Geometry check sheet. Reference: drawing and pictorial views, mm from the part's lowest x, y, z. Give positions to 0.01 mm unless a question says otherwise; leave off trailing zeros. Order: outer loops, then holes, each group sorted by start corner. A loop starts at its lowest first (then second) coordinate and runs counter-clockwise, first axis right, second up.
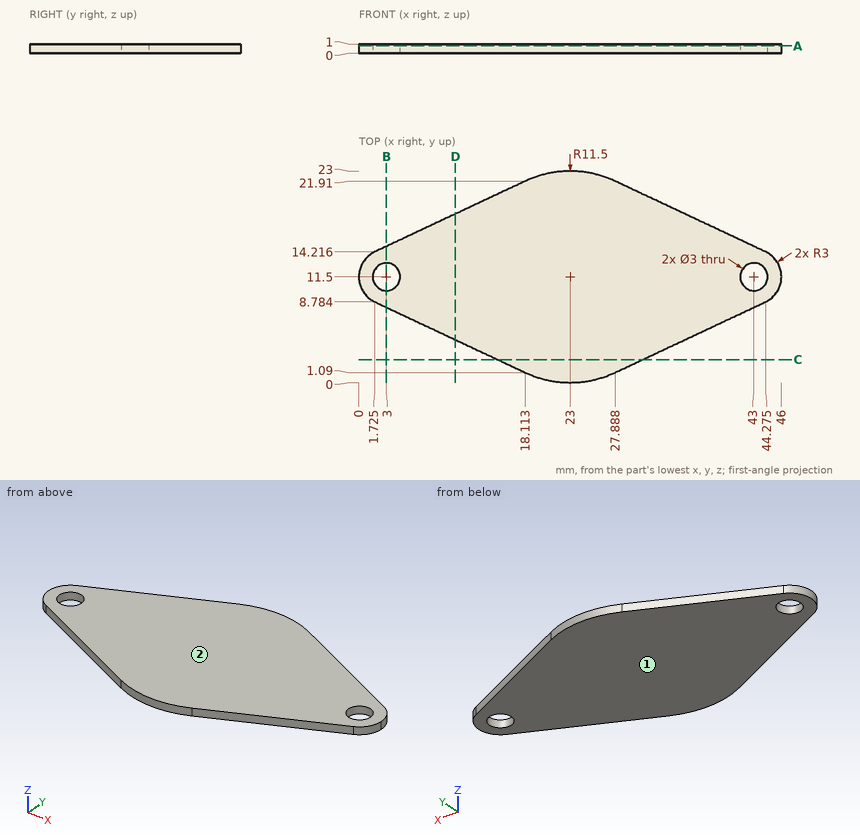
1) Depth check by flat-ended pin: pin 1 Ø3.5 at (x, y) = (3, 11.5) entering from -Z. Enter the tip coordinate at first touch or a pass-through.
Recorded:
pin 1: stops at z = 0
2) Section check D-D, the plane x = 10.5. Record the cut outline in (y, z) (1 decimal).
Recorded:
outline: (4.7, 0) - (18.3, 0) - (18.3, 1) - (4.7, 1) - close
3) Draft check along Z on the marked faces 1 and 2. Enter one of: +Z half, -Z half, draft (parallel to the pull), parting line (faces both ways), or undercut.
Recorded:
face 1: -Z half
face 2: +Z half
4) Section check C-C, the plane y = 2.5. Record the cut outline in (x, z).
Recorded:
outline: (15.11, 0) - (30.89, 0) - (30.89, 1) - (15.11, 1) - close
5) Material ranges on L1, parallel to X at y = 12, z = 0.5 (1 decimal); L2, parallel to X at y = 11.75, z = 0.5; L3, parallel to Y at x = 3, z = 0.75 (1 decimal), recorded low to high.
Recorded:
L1: x = 0 to 1.6, 4.4 to 41.6, 44.4 to 46
L2: x = 0.01 to 1.52, 4.48 to 41.52, 44.48 to 45.99
L3: y = 8.2 to 10, 13 to 14.8
6) Section check A-A, the plane z = 0.8. Record the cut outline in (x, y) (1 decimal).
Recorded:
outline: (1.7, 8.8) - (18.1, 1.1) arc R11.5 ccw to (27.9, 1.1) - (44.3, 8.8) arc R3 ccw to (46, 11.5) arc R3 ccw to (44.3, 14.2) - (27.9, 21.9) arc R11.5 ccw to (18.1, 21.9) - (1.7, 14.2) arc R3 ccw to start; hole circle Ø3 at (3, 11.5); hole circle Ø3 at (43, 11.5)
7) Section check B-B, the plane x = 3. Record the cut outline in (y, z) (1 decimal).
Recorded:
outline: (8.2, 0) - (10, 0) - (10, 1) - (8.2, 1) - close; (13, 0) - (14.8, 0) - (14.8, 1) - (13, 1) - close
